Geometry check sheet. Reference: the model listing, model coordinates, mm. A direction names the side the tool comes from. Round coordinates to 2 decimals unless told otherwise and drop trailing zeros. Loops run counter-clockwise (first coordinate to the right, second up) from the corner with the lowest first, then second, coordinate; pieces in that order, holes last.
Autodesk Inventor part; units mm, degrees
ref_plane "YZ Plane" through (0, 0, 0) normal (1, 0, 0) x (0, 1, 0)
ref_plane "XZ Plane" through (0, 0, 0) normal (0, 1, 0) x (-1, 0, 0)
ref_plane "XY Plane" through (0, 0, 0) normal (0, 0, 1) x (1, 0, 0)
sketch "Sketch1" plane through (0, 0, 0) normal (0, 1, 0) x (-1, 0, 0)
  line L0 (0, 0) -> (-11, 0)
  line L1 (-11, 0) -> (-11, -17)
  line L2 (-11, -17) -> (0, -17)
  line L3 (0, -17) -> (0, 0)
  circle A0 centre (-5.5, 0) radius 3
  circle A1 centre (-5.5, -17) radius 3
  circle A2 centre (-5.5, 0) radius 1.5
  circle A3 centre (-5.5, -17) radius 1.5
  circle A4 centre (-5.5, -17) radius 3
  circle A5 centre (-5.5, -17) radius 1.5
  circle A6 centre (-5.5, 0) radius 1.5
  circle A7 centre (-5.5, 0) radius 3
  point P0 (-8.5, -17)
  point P1 (-2.5, -17)
  point P2 (-2.5, 0)
  point P3 (-8.5, 0)
  dimension "d0" = 11
  dimension "d1" = 17
  dimension "d2" = 6
  dimension "d3" = 6
  dimension "d6" = 3
  dimension "d7" = 3
extrude "Extrusion1" add sketch "Sketch1" along normal blind 2
sketch "Sketch2" plane through (0, 2, 0) normal (0, 1, 0) x (1, 0, 0)
  point P0 (0, 0)
sketch "Sketch3" plane through (0, 0, 0) normal (0, -1, 0) x (1, 0, 0)
  point P0 (0, 0)
sketch "Sketch4" plane through (0, 0, 0) normal (0, -1, 0) x (1, 0, 0)
  arc A0 (8.5, 0) -> (2.5, 0) centre (5.5, 0) ccw
  circle A1 centre (5.5, 0) radius 1.5
  arc A2 (2.5, -17) -> (8.5, -17) centre (5.5, -17) ccw
  circle A3 centre (5.5, -17) radius 1.5
  circle A4 centre (5.5, -17) radius 1.5
  circle A5 centre (5.5, 0) radius 1.5
  point P0 (0, 0)
  dimension "d8" = 3
  dimension "d9" = 3
hole "Hole1" at (5.5, 0, 0) at (5.5, 0, -17) direction (0, 1, 0) diameter 3 end through all
properties part number "przykrywka"
1) Gauge pin test, flat end, axial feed: pin 1 (1 mm diameter, centred on x = 10, y = 0.5, fed in from +Z). Record the tip position at first contact, or that the pin passes through.
Report:
pin 1: stops at z = 0
2) Scan lines: line 1 along Z through (x, y) = (5.25, 0.95); line 2 along Z through (x, y) = (4.75, 0.65); line 3 along Z through (x, y) = (9.5, 0.7). Record each from-to range of solid material in increasing order.
Report:
line 1: z = -19.99 to -18.48, -15.52 to -1.48, 1.48 to 2.99
line 2: z = -19.9 to -18.3, -15.7 to -1.3, 1.3 to 2.9
line 3: z = -17 to 0
3) Mould release check, pull along X, two halves, no side actions. Record for faces 6 (the face through (0, 1, -9)), 7 (the face through (5.6, 1, 3)), 8 (the face through (10, 1, 0)), 9 (the face through (4.235, 1.014, -0.806)): +X half, -X half, draft (parallel to the pull), parting line (faces both ways), or undercut.
Report:
face 6: -X half
face 7: parting line
face 8: draft
face 9: undercut
4) Sectioned sample at A-A, the plane z = -16. Record the cut outline in (x, y), then the cut area to 3 significant figures.
Report:
outline: (0, 0) - (4.38, 0) - (4.38, 2) - (0, 2) - close; (6.62, 0) - (11, 0) - (11, 2) - (6.62, 2) - close
area: 17.5 mm2
5) Sectioned sample at D-D, the plane x = 2.25. Record the cut outline in (y, z).
Report:
outline: (0, -17) - (2, -17) - (2, 0) - (0, 0) - close
6) Access from +Z, -Z, +X, -X, +Y, -Y to the whole of each face (thin tool, end or side, straight path). Record for faces 1 (the face through (5.43, 1.01, -15.5)), 2 (the face through (1, 1, -17)), 3 (the face through (1, 1, 0)), 4 (the face through (10, 1, -17)), 5 (the face through (11, 1, -8)).
Report:
face 1: +Y, -Y
face 2: -Z, -X, +Y, -Y
face 3: +Z, -X, +Y, -Y
face 4: -Z, +X, +Y, -Y
face 5: +Z, -Z, +X, +Y, -Y
7) Sectioned sample at C-C, the plane y = 1.15. Record the cut outline in (x, z), then the cut area to 3 significant figures.
Report:
outline: (0, -17) - (2.5, -17) arc R3 ccw to (8.5, -17) - (11, -17) - (11, 0) - (8.5, 0) arc R3 ccw to (2.5, 0) - (0, 0) - close; hole circle Ø3 at (5.5, -17); hole circle Ø3 at (5.5, 0)
area: 201 mm2
8) Sectioned sample at B-B, the plane x = 5.5. Record the cut outline in (y, z).
Report:
outline: (0, -20) - (2, -20) - (2, -18.5) - (0, -18.5) - close; (0, -15.5) - (2, -15.5) - (2, -1.5) - (0, -1.5) - close; (0, 1.5) - (2, 1.5) - (2, 3) - (0, 3) - close
